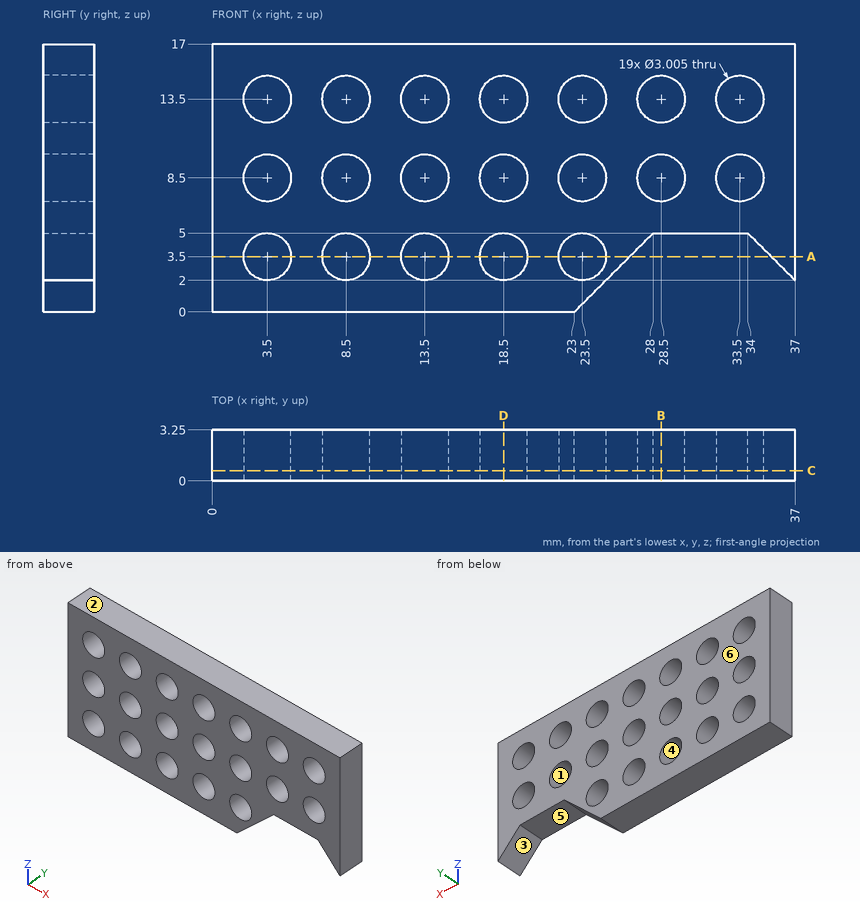
Geometry check sheet. Reference: drawing and pictorial views, mm from the part's lowest x, y, z. A direction names the side the tool comes from. Round coordinates to 2 decimals unless told otherwise and drop trailing zeros. Write each loop counter-clockwise with the first axis right and the second up, starting at its lowest first coordinate (ties: lowest second). Pieces come first, ordered by that corner, then holes.
Item 1: Go/stop test with flat-tipped pins: pin 1 Ø2.5 at (x, z) = (13.5, 8.5) entering from +Y; pin 2 Ø1.6 at (x, y) = (31, 2.5) entering from -Z. Record where each tip stops, or that it passes through.
Determined:
pin 1: passes through
pin 2: stops at z = 5
Item 2: Section check B-B (x = 28.5). Record the boundary of the cut face in (y, z).
Determined:
outline: (0, 5) - (3.25, 5) - (3.25, 7) - (0, 7) - close; (0, 10) - (3.25, 10) - (3.25, 12) - (0, 12) - close; (0, 15) - (3.25, 15) - (3.25, 17) - (0, 17) - close
Item 3: Section check D-D (x = 18.5). Record the boundary of the cut face in (y, z).
Determined:
outline: (0, 0) - (3.25, 0) - (3.25, 2) - (0, 2) - close; (0, 5) - (3.25, 5) - (3.25, 7) - (0, 7) - close; (0, 10) - (3.25, 10) - (3.25, 12) - (0, 12) - close; (0, 15) - (3.25, 15) - (3.25, 17) - (0, 17) - close
Item 4: Material ranges on line 1 along Z through (x, y) = (12.5, 1.85); line 2 along Z through (x, y) = (33.5, 1.15); line 3 along Z through (x, y) = (23.5, 2.05), recorded low to high.
Determined:
line 1: z = 0 to 2.38, 4.62 to 7.38, 9.62 to 12.38, 14.62 to 17
line 2: z = 5 to 7, 10 to 12, 15 to 17
line 3: z = 0.5 to 2, 5 to 7, 10 to 12, 15 to 17
Item 5: Access from +Z, -Z, +X, -X, +Y, -Y to the whole of each face (thin tool, end or side, straight path). Record for the marked faces 5 and 6.
Determined:
face 5: -Z, +Y, -Y
face 6: +Z, -Z, +X, -X, +Y
Item 6: Section check A-A (z = 3.5). Record the boundary of the cut face in (x, y), plus the area to 3 significant figures.
Determined:
outline: (0, 0) - (2, 0) - (2, 3.25) - (0, 3.25) - close; (5, 0) - (7, 0) - (7, 3.25) - (5, 3.25) - close; (10, 0) - (12, 0) - (12, 3.25) - (10, 3.25) - close; (15, 0) - (17, 0) - (17, 3.25) - (15, 3.25) - close; (20, 0) - (22, 0) - (22, 3.25) - (20, 3.25) - close; (25, 0) - (26.5, 0) - (26.5, 3.25) - (25, 3.25) - close; (35.5, 0) - (37, 0) - (37, 3.25) - (35.5, 3.25) - close
area: 42.2 mm2
Item 7: Section check C-C (y = 0.65). Give the number of separate pieces and of enclosed holes in the cut face, plus the area to 3 significant figures.
Determined:
separate pieces: 1
enclosed holes: 19
area: 441 mm2
Item 8: Mould release check, pull along Z, two halves, no side actions. Record for the marked faces 1, 2, 3 and 4: +Z half, -Z half, draft (parallel to the pull), parting line (faces both ways), or undercut.
Determined:
face 1: undercut
face 2: +Z half
face 3: -Z half
face 4: undercut
